Can you work these out from the drawing? Everything is in mm from the part's minimum corner. A direction names the side the tool comes from. Coordinates: 2 decimals unless noted, no trailing zeros. Write each loop counter-clockwise with the first axis right and the second up, starting at its lowest first coordinate (ties: lowest second). Pieces come first, ordered by that corner, then holes. Notation, with made-up numbers: M 8,-11 L 13,-11 A8 cw 13,4 Z; hole C -7.5,-17 d8. An arc over 180 degrees is marked long. Use one line per item in the form item = value. Start each with the question number.
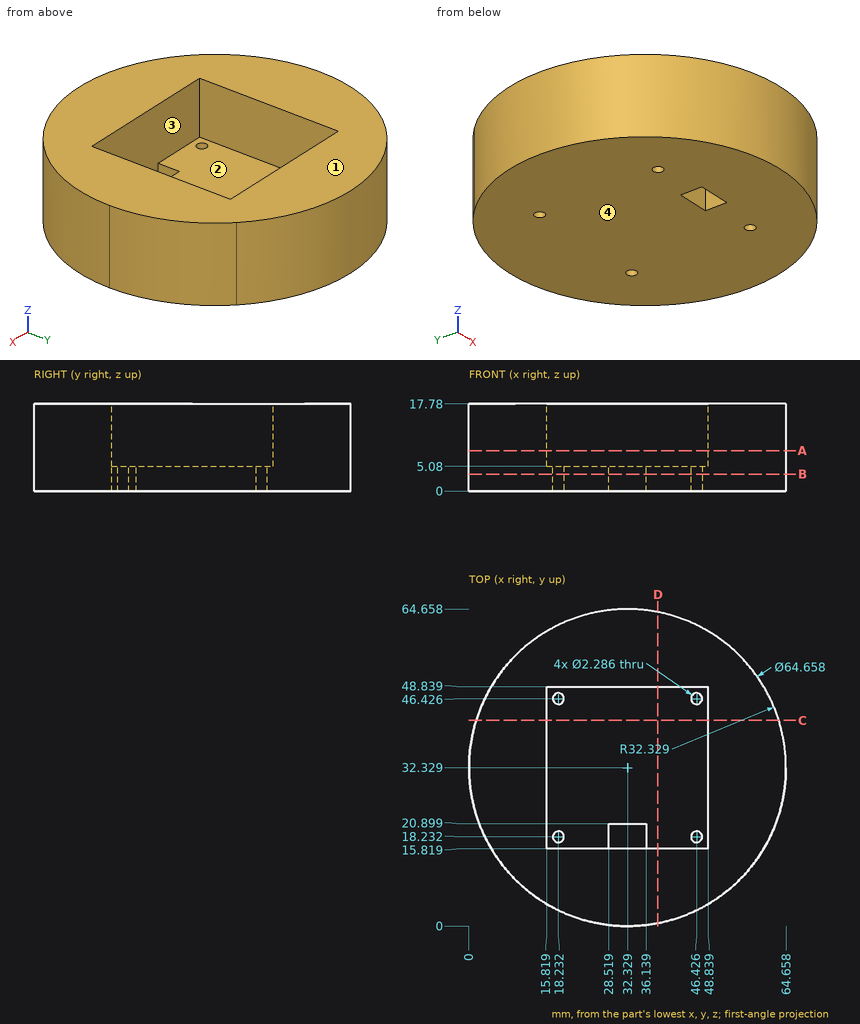
1) Suppose I cut it at C-C on y = 42. Please give me the cut outline in (x, z).
2) Suppose I cut it at D-D on x = 38.5. Please give me the cut outline in (y, z).
3) Please list where these lines run through material, in increasing order: line 1 (Z direction, x = 40.5, y = 23.5); line 2 (X direction, y = 25, z = 7); line 3 (Y direction, x = 40.5, z = 9.5).
4) If we mould it in two halves opening along X, with no side actions, what happens to the marked faces 3 and 4? For each: +X half, -X half, draft (parallel to the pull), parting line (faces both ways), or undercut.
5) Which directions (+Z, -Z, +X, -X, +Y, -Y) give clear straight access to the entire face, cutting with the end or side of a thin tool? Please do the marked faces 1 and 2.
6) Suppose I cut it at A-A on z = 8.25. Please give me the cut outline in (x, y).
7) Will these pins go through, and if not, where does the flat tip stop? pin 1 Ø2.5 at (x, z) = (33.5, 2.5) entering from -Y; pin 2 Ø1.5 at (y, z) = (17.5, 1.5) entering from -X; pin 3 Ø5.5 at (y, z) = (17.5, 3) entering from +X; pin 4 Ø1.4 at (x, y) = (46.43, 18.23) entering from +Z.
8) Suppose I cut it at B-B on z = 3.5. Please give me the cut outline in (x, y) (3 decimals), and give its area (3 significant figures).
Computed values:
q1.outline = M 1.48,0 L 63.18,0 L 63.18,17.78 L 48.84,17.78 L 48.84,5.08 L 15.82,5.08 L 15.82,17.78 L 1.48,17.78 Z
q2.outline = M 0.59,0 L 64.06,0 L 64.06,17.78 L 48.84,17.78 L 48.84,5.08 L 15.82,5.08 L 15.82,17.78 L 0.59,17.78 Z
q3.line_1 = 0 to 5.08
q3.line_2 = 0.84 to 15.82, 48.84 to 63.82
q3.line_3 = 1.05 to 15.82, 48.84 to 63.61
q4.face_3 = undercut
q4.face_4 = draft
q5.face_1 = +Z, +X, -X, +Y, -Y
q5.face_2 = +Z
q6.outline = C 32.33,32.33 d64.66; hole M 15.82,15.82 L 48.84,15.82 L 48.84,48.84 L 15.82,48.84 Z
q7.pin_1 = 0
q7.pin_2 = 3.23
q7.pin_3 = 62.32
q7.pin_4 = through
q8.outline = C 32.329,32.329 d64.658; hole C 18.232,18.232 d2.286; hole C 18.232,46.426 d2.286; hole M 28.519,15.819 L 36.139,15.819 L 36.139,20.899 L 28.519,20.899 Z; hole C 46.426,18.232 d2.286; hole C 46.426,46.426 d2.286
q8.area = 3,230 mm²
